Could you check a few things on this model? Use its own coordinates, in mm. A direction names the side the tool comes from. Give positions to 0.01 mm unless a question says otherwise; leave off trailing zeros. Order: outer loops, then holes, each group sorted by start corner. A loop starts at its lowest first (then second) coordinate and runs counter-clockwise, first axis right, second up. Notation, with made-up numbers: (68, 38.5) -> (80, 38.5) arc R13 cw to (80, 45.5) -> close; hole circle Ø9 at (44.5, -40). An arc over 180 degrees is marked (long way). Answer as CSV lines item,"result". Start each with the question number.
(1) I want a section at C-C (x = 40). Please give me the cut outline in (y, z).
(2) Will these pins go through, and if not, where does the flat tip stop? pin 1 Ø5 at (x, z) = (40, 0) entering from -Y; pin 2 Ø0.6 at (y, z) = (-1.5, 36) entering from +X.
(3) On a 3-axis mill with a long thin cutter (end or side, diameter ignored), from which of +Z, -Z, +X, -X, +Y, -Y can I reach the whole of each face in a straight line? I mean faces 1 (the face through (10, -1, 31)), 2 (the face through (-9, -1, 48)). Say none if no direction works.
(4) I need wall thicknesses on L1, parallel to X at y = -0.8, z = 0; L2, parallel to X at y = -1.2, z = 40; L3, parallel to Z at x = 43, y = -1.1. Which ranges of each line are inside material? Lowest first, please.
(5) I want a section at A-A (z = 20). Please give me the cut outline in (x, y).
(6) I want a section at D-D (y = -0.4). Please give me the cut outline in (x, z), plus the area to 3 significant figures.
(7) I want a section at B-B (x = 0). Please give me the cut outline in (y, z).
(8) We'd pull the mould along X, two halves only. Please class faces 3 (the face through (50, -1, 0)), 4 (the face through (-0.8, -0.99, 21.94)), 5 (the face through (14, -2, 6)): released by +X, released by -X, zero draft, split by the parting line, or undercut.
```python
from build123d import *

# Parameters (mm, degrees)
SKETCH1_R          = 2.1
BASE_FLANGE1_DEPTH = 2
FILLET_SHAPE_R     = 5
CHAMFER2_SIZE      = 5
FILLET2_R          = 5


# Sheet-metal steps are written as plain solids
with BuildPart() as part:
    # Sketch1 → Base-Flange1 (new body)
    with BuildSketch(Plane(origin=(0, 0, 0), x_dir=(1, 0, 0), z_dir=(0, 1, 0))):
        Polygon((-10, 10), (50, 10), (50, -10), (10, -10), (10, -50), (-10, -50), align=None)
        with Locations(Location((0, 0, 0), (0, 0, 270))):
            Circle(SKETCH1_R, mode=Mode.SUBTRACT)
        with Locations(Location((20, 0, 0), (0, 0, 270))):
            Circle(SKETCH1_R, mode=Mode.SUBTRACT)
        with Locations(Location((40, 0, 0), (0, 0, 270))):
            Circle(SKETCH1_R, mode=Mode.SUBTRACT)
        with Locations(Location((0, -20, 0), (0, 0, 270))):
            Circle(SKETCH1_R, mode=Mode.SUBTRACT)
        with Locations(Location((0, -40, 0), (0, 0, 270))):
            Circle(SKETCH1_R, mode=Mode.SUBTRACT)
    extrude(amount=-BASE_FLANGE1_DEPTH)

    # Fillet_Shape
    fillet_shape_edges = [part.edges().sort_by_distance(p)[0] for p in [
        (10, -1, 50),
        (-10, -1, 50),
        (-10, -1, -10),
        (50, -1, -10),
        (50, -1, 10),
    ]]
    fillet(fillet_shape_edges, radius=FILLET_SHAPE_R)

    # Chamfer2
    chamfer2_edges = [part.edges().sort_by_distance(p)[0] for p in [
        (10, -1, 10),
    ]]
    chamfer(chamfer2_edges, length=CHAMFER2_SIZE)

    # Fillet2
    fillet2_edges = [part.edges().sort_by_distance(p)[0] for p in [
        (10, -1, 15),
        (15, -1, 10),
    ]]
    fillet(fillet2_edges, radius=FILLET2_R)


solid = part.part
```
Final values:
1,outline,"(-2, -10) -> (0, -10) -> (0, -2.1) -> (-2, -2.1) -> close; (-2, 2.1) -> (0, 2.1) -> (0, 10) -> (-2, 10) -> close"
2,pin 1,"y = -2"
2,pin 2,"x = 10"
3,face 1,"+Z, +X, +Y, -Y"
3,face 2,"+Z, -X, +Y, -Y"
4,L1,"-10 to -2.1, 2.1 to 17.9, 22.1 to 37.9, 42.1 to 50"
4,L2,"-10 to -2.1, 2.1 to 10"
4,L3,"-10 to 10"
5,outline,"(-10, -2) -> (-2.1, -2) -> (-2.1, 0) -> (-10, 0) -> close; (2.1, -2) -> (10, -2) -> (10, 0) -> (2.1, 0) -> close"
6,outline,"(-10, -5) arc R5 ccw to (-5, -10) -> (45, -10) arc R5 ccw to (50, -5) -> (50, 5) arc R5 ccw to (45, 10) -> (17.07, 10) arc R5 cw to (13.54, 11.46) -> (11.46, 13.54) arc R5 cw to (10, 17.07) -> (10, 45) arc R5 ccw to (5, 50) -> (-5, 50) arc R5 ccw to (-10, 45) -> close; hole circle Ø4.2 at (0, 0); hole circle Ø4.2 at (0, 20); hole circle Ø4.2 at (0, 40); hole circle Ø4.2 at (20, 0); hole circle Ø4.2 at (40, 0)"
6,area,"1,920 mm²"
7,outline,"(-2, -10) -> (0, -10) -> (0, -2.1) -> (-2, -2.1) -> close; (-2, 2.1) -> (0, 2.1) -> (0, 17.9) -> (-2, 17.9) -> close; (-2, 22.1) -> (0, 22.1) -> (0, 37.9) -> (-2, 37.9) -> close; (-2, 42.1) -> (0, 42.1) -> (0, 50) -> (-2, 50) -> close"
8,face 3,"released by +X"
8,face 4,"undercut"
8,face 5,"zero draft"
